```python
from build123d import *

# Parameters (mm, degrees)
SWEEP1_PROFILE_R   = 16.5
SKETCH10_W         = 17
SKETCH10_H         = 17
CUT_EXTRUDE1_DEPTH = 25
SKETCH11_R         = 3.5
CUT_EXTRUDE2_DEPTH = 13
SKETCH12_R         = 5
CUT_EXTRUDE3_DEPTH = 13


with BuildPart() as part:
    # Sweep1: sweep along a path in Sketch1
    with BuildLine(Plane(origin=(0, 0, 0), x_dir=(0, 0, -1), z_dir=(1, 0, 0))) as sweep1_path:
        Line((81.472527473, -41.846153846), (81.472527473, -36.846153846))
        ThreePointArc((81.472527473, -36.846153846), (74.150197002, -19.168484316), (56.472527473, -11.846153846))
        Line((56.472527473, -11.846153846), (-113.527472527, -11.846153846))
        ThreePointArc((-113.527472527, -11.846153846), (-131.205142057, -19.168484316), (-138.527472527, -36.846153846))
        Line((-138.527472527, -36.846153846), (-138.527472527, -46.846153846))
    # Sweep1 profile (on start of the path) → Sweep1 (sweep)
    with BuildSketch(Plane(origin=(0, -41.846153846, -81.472527473), x_dir=(0, 0, 1), z_dir=(0, 1, 0))):
        Circle(SWEEP1_PROFILE_R)
    sweep(path=sweep1_path.line)

    # Sketch10 → Cut-Extrude1 (cut)
    with BuildSketch(Plane.XZ.offset(46.846153846)):
        with Locations((0, 138.527472527)):
            Rectangle(SKETCH10_W, SKETCH10_H)
    extrude(amount=-CUT_EXTRUDE1_DEPTH, mode=Mode.SUBTRACT)

    # Sketch11 → Cut-Extrude2 (cut)
    with BuildSketch(Plane.XZ.offset(21.846153846)):
        with Locations(Location((0, 138.527472527, 0), (0, 0, 270))):
            Circle(SKETCH11_R)
    extrude(amount=-CUT_EXTRUDE2_DEPTH, mode=Mode.SUBTRACT)

    # Sketch12 → Cut-Extrude3 (cut)
    with BuildSketch(Plane.XZ.offset(8.846153846)):
        with Locations(Location((0, 138.527472527, 0), (0, 0, 270))):
            Circle(SKETCH12_R)
    extrude(amount=-CUT_EXTRUDE3_DEPTH, mode=Mode.SUBTRACT)


solid = part.part
```
Here's how the part is built. I have some questions about the finished solid (model axes, mm). A direction names the side the tool comes from. Give positions to 0.01 mm unless a question says otherwise; leave off trailing zeros. Write each loop counter-clockwise with the first axis right and the second up, starting at its lowest first coordinate (ties: lowest second). Pieces come first, ordered by that corner, then holes. Notation, with made-up numbers: (-27, 30) -> (0, 30) arc R15 cw to (0, 47) -> close; hole circle Ø1 at (8, -30.5). An arc over 180 degrees is marked (long way). Write each question's results on one line, items separated by ' | '.
Item 1: Suppose I cut it at B-B on x = -14. Write out the boundary of the cut face in (y, z).
Output:
outline: (-46.85, 129.8) -> (-36.85, 129.8) arc R16.27 cw to (-20.58, 113.53) -> (-20.58, -56.47) arc R16.27 cw to (-36.85, -72.74) -> (-41.85, -72.74) -> (-41.85, -90.2) -> (-36.85, -90.2) arc R33.73 ccw to (-3.11, -56.47) -> (-3.11, 113.53) arc R33.73 ccw to (-36.85, 147.26) -> (-46.85, 147.26) -> close
Item 2: On a 3-axis mill with a long thin cutter (end or side, diameter ignored), from which of +Z, -Z, +X, -X, +Y, -Y can I reach the whole of each face in a straight line? I mean faces 1 (the face through (4.956, -39.311, -65.734)), 2 (the face through (1.502, -5.653, 133.758)), 3 (the face through (0, -46.846, 128)). Say none if no direction works.
Output:
face 1: -Y | face 2: +Y | face 3: +Z, -Z, +X, -X, -Y
Item 3: We'd pull the mould along X, two halves only. Please class faces 4 (the face through (-10.04, 1.25, 29.72)), 5 (the face through (0, -41.846, -82)), 6 (the face through (-0.1, -21.846, 142.4)): pulls with the +X half, pulls with the -X half, needs draft (parallel to the pull), parting line crosses it, or undercut.
Output:
face 4: parting line crosses it | face 5: needs draft | face 6: undercut
Item 4: Suppose I cut it at C-C on z = -4.5. Write out the boundary of the cut face in (x, y).
Output:
outline: circle Ø33 at (0, -11.85)
Item 5: For pin 1 Ø8 at (x, z) = (0, 138.53) entering from -Y; pin 2 Ø2 at (x, y) = (-10, -37.5) entering from +Z; pin 3 Ø5 at (x, y) = (13, -15) entering from +Z, each with a flat end and sliding along its axis, tell me the tip position at first contact or that it passes through.
Output:
pin 1: stops at y = -21.85 | pin 2: stops at z = 152.36 | pin 3: stops at z = 144.8
Item 6: If I drill on L1, parallel to Z at x = -4, y = -32; L2, parallel to Z at x = -0.5, y = -33.5; L3, parallel to Z at x = 10, y = -30, over which ranges is the centre line in solid material (lowest first)?
Output:
L1: z = -97.19 to -64.05, 121.1 to 130.03, 147.03 to 154.25 | L2: z = -97.83 to -64.29, 121.35 to 130.03, 147.03 to 154.88 | L3: z = -93.98 to -66.18, 123.23 to 151.03
Item 7: Suppose I cut it at A-A on x = 0. Write out the boundary of the cut face in (y, z), plus the area to 3 significant figures.
Output:
outline: (-46.85, 122.03) -> (-36.85, 122.03) arc R8.5 cw to (-28.35, 113.53) -> (-28.35, -56.47) arc R8.5 cw to (-36.85, -64.97) -> (-41.85, -64.97) -> (-41.85, -97.97) -> (-36.85, -97.97) arc R41.5 ccw to (4.65, -56.47) -> (4.65, 113.53) arc R41.5 ccw to (-0.48, 133.53) -> (-8.85, 133.53) -> (-8.85, 135.03) -> (-21.85, 135.03) -> (-21.85, 130.03) -> (-46.85, 130.03) -> close; (-46.85, 147.03) -> (-21.85, 147.03) -> (-21.85, 142.03) -> (-8.85, 142.03) -> (-8.85, 143.53) -> (-8.17, 143.53) arc R41.5 ccw to (-36.85, 155.03) -> (-46.85, 155.03) -> close | area: 8,130 mm^2
